Verification items for this drawing (mm, ordinates from the low corner). A direction names the side the tool comes from. Coordinates: 2 decimals unless noted, no trailing zeros. Order: outer loops, then holes, each group sorted by start corner. A loop starts at its lowest first (then second) coordinate and runs counter-clockwise, first axis right, second up.
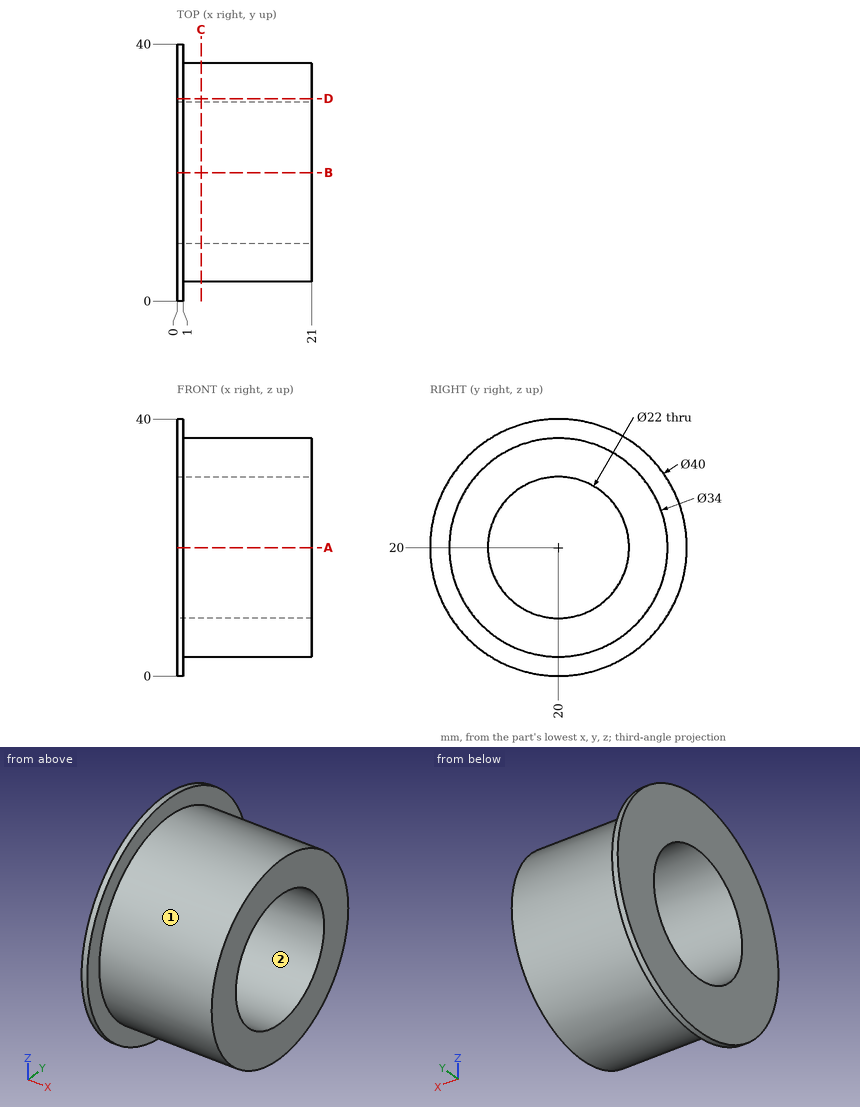
Item 1: Thickness scan on line 1 along Y through (x, z) = (9.5, 20); line 2 along Z through (x, y) = (16.75, 23.5); line 3 along Y through (x, z) = (11.5, 18.5). Record the ranges inside material, lowest first.
Item 2: Sectioned sample at A-A (z = 20). Record the cut outline in (x, y).
Item 3: Sectioned sample at D-D (y = 31.5). Record the cut outline in (x, z), and give its area (3 significant figures).
Item 4: Tool access check on the marked faces 1 and 2. Record the directions out of +Z, -Z, +X, -X, +Y, -Y that give a thin tool (end or side, any length) a straight path to the whole face; none if there is none.
Item 5: Sectioned sample at C-C (x = 3.75). Record the cut outline in (y, z).
Item 6: Depth check by flat-ended pin: P1, Ø5, axis at x = 10, z = 8.5, coming from the -Y side; P2, Ø5, axis at x = 8, y = 24.5, coming from the +Z side; P3, Ø1.5, axis at x = 15, z = 11, coming from the +Y side. Enter the tip coordinate at first touch or a pass-through.
Geometry check:
1. line 1: y = 3 to 9, 31 to 37
1. line 2: z = 3.36 to 9.57, 30.43 to 36.64
1. line 3: y = 3.07 to 9.1, 30.9 to 36.93
2. outline: (0, 0) - (1, 0) - (1, 3) - (21, 3) - (21, 9) - (0, 9) - close; (0, 31) - (21, 31) - (21, 37) - (1, 37) - (1, 40) - (0, 40) - close
3. outline: (0, 3.64) - (1, 3.64) - (1, 7.48) - (21, 7.48) - (21, 32.52) - (1, 32.52) - (1, 36.36) - (0, 36.36) - close
3. area: 534 mm2
4. face 1: +X
4. face 2: +X, -X
5. outline: circle Ø34 at (20, 20); hole circle Ø22 at (20, 20)
6. P1: stops at y = 5.58
6. P2: stops at z = 36.88
6. P3: stops at y = 34.86
